from build123d import *

# Parameters (mm, degrees)
ESQUISSE2_R             = 1.692758077
BOSS_EXTRU_1_DEPTH      = 15
ESQUISSE3_R             = 4
BOSS_EXTRU_2_DEPTH      = 2.5
ESQUISSE4_R             = 1.25
ENL_V_MAT_EXTRU_1_DEPTH = 5


with BuildPart() as part:
    # Esquisse1 → Révolution1 (revolve)
    with BuildSketch(Plane.XY):
        Polygon((0, 0), (12.15, 0), (12.15, 2.5), (12.5, 2.5), (12.5, 54.5), (13, 54.5), (13, 93.5), (7, 93.5), (7, 96), (2.5, 96), (2.5, 110), (0, 110), align=None)
    revolve(axis=Axis((0, 0, 0), (0, 1, 0)))

    # Esquisse2 → Boss.-Extru.1 (add)
    with BuildSketch(Plane.XZ):
        Circle(ESQUISSE2_R)
    extrude(amount=BOSS_EXTRU_1_DEPTH)

    # Esquisse3 → Boss.-Extru.2 (add)
    with BuildSketch(Plane.XZ):
        Circle(ESQUISSE3_R)
    extrude(amount=BOSS_EXTRU_2_DEPTH)

    # Esquisse4 → Enlèv. mat.-Extru.1 (cut)
    with BuildSketch(Plane(origin=(0, 93.5, 0), x_dir=(1, 0, 0), z_dir=(0, 1, 0))):
        with Locations((0, 10)):
            Circle(ESQUISSE4_R)
        with Locations((10, 0)):
            Circle(ESQUISSE4_R)
        with Locations((0, -10)):
            Circle(ESQUISSE4_R)
        with Locations((-10, 0)):
            Circle(ESQUISSE4_R)
    extrude(amount=-ENL_V_MAT_EXTRU_1_DEPTH, mode=Mode.SUBTRACT)


solid = part.part
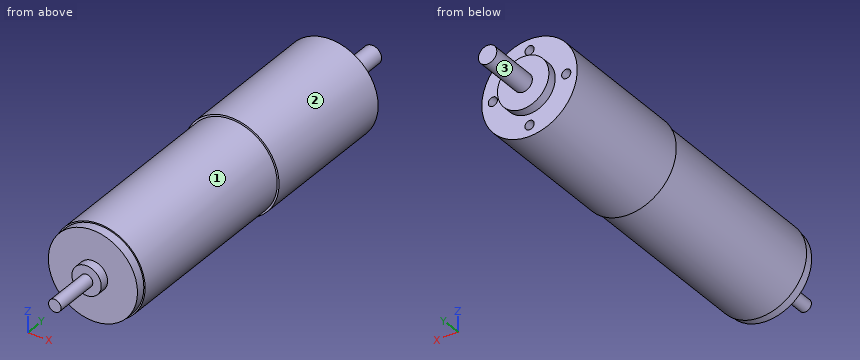
Input: part model. Units: mm. Frame: model coordinates. Face numbers are marked on the shaded views. A direction names the side the tool comes from. Round coordinates to 2 decimals unless told otherwise and drop trailing zeros. Order: outer loops, then holes, each group sorted by start corner. A loop starts at its lowest first (then second) coordinate and runs counter-clockwise, first axis right, second up.
1. Set-up query: the marked faces 1, 2 and 3. Return all of +Z, -Z, +X, -X, +Y, -Y with unobstructed straight access to the full face (end or side cutting, diameter ignored); none if empty.
The answers:
face 1: -Y
face 2: +Y, -Y
face 3: +Y
2. Pin query (flat end, axial travel): P1, Ø2, axis at y = 50, z = 5.5, coming from the -X side; P2, Ø5, axis at y = 22, z = 7.5, coming from the +X side; P3, Ø2, axis at x = 0, z = -10.5, coming from the +Y side. Return the tip coordinate at first contact, or that it passes through.
The answers:
P1: stops at x = -11.66
P2: stops at x = 11.46
P3: stops at y = 93.5
3. Material intervals for line 1 (X direction, y = 89.95, z = 0); line 2 (X direction, y = 90.25, z = 10), sorted ascending.
The answers:
line 1: x = -13 to -11.25, -8.75 to 8.75, 11.25 to 13
line 2: x = -8.31 to -1.25, 1.25 to 8.31
4. Cut plane A-A, the plane z = 5.5. Output: boundary loops of the cut face in (x, y).
The answers:
outline: (-11.78, 54.5) - (-11.22, 54.5) - (-11.22, 2.5) - (-10.83, 2.5) - (-10.83, 0) - (10.83, 0) - (10.83, 2.5) - (11.22, 2.5) - (11.22, 54.5) - (11.78, 54.5) - (11.78, 93.5) - (4.33, 93.5) - (4.33, 96) - (-4.33, 96) - (-4.33, 93.5) - (-11.78, 93.5) - close
5. Cut plane C-C, the plane y = 52. Output: boundary loops of the cut face in (x, z), then the cut area to 3 significant figures.
The answers:
outline: circle Ø25 at (0, 0)
area: 491 mm2
6. Cut plane B-B, the plane x = 10. Output: boundary loops of the cut face in (y, z), then the cut area to 3 significant figures.
The answers:
outline: (0, -6.9) - (2.5, -6.9) - (2.5, -7.5) - (54.5, -7.5) - (54.5, -8.31) - (93.5, -8.31) - (93.5, -1.25) - (88.5, -1.25) - (88.5, 1.25) - (93.5, 1.25) - (93.5, 8.31) - (54.5, 8.31) - (54.5, 7.5) - (2.5, 7.5) - (2.5, 6.9) - (0, 6.9) - close
area: 1,450 mm2
